Model file for the job. Use its own axes, mm. Face numbers are marked on the shaded views. Give positions to 0.01 mm unless a question says otherwise; leave off trailing zeros. Loops run counter-clockwise (first coordinate to the right, second up) from the corner with the lowest first, then second, coordinate; pieces in that order, holes last. Notation, with made-up numbers: M 36,19 L 94,19 A17 ccw 94,46 Z; hole C 24,63 d3. An arc over 180 degrees is marked long. Answer in a Markdown table with one row per item.
```python
from build123d import *

# Parameters (mm, degrees)
F0_R     = 19.08734
F0_R_2   = 10.668378
F1_DEPTH = 25.4


with BuildPart() as f1:
    # F0 (on Front) → F1 (new body)
    with BuildSketch(Plane.XZ):
        with BuildLine():
            Line((115.265532, 26.16193), (3.586851, 36.99093))
            ThreePointArc((3.586851, 36.99093), (-37.164423, 0), (3.586851, -36.99093))
            Line((3.586851, -36.99093), (115.265532, -26.16193))
            ThreePointArc((115.265532, -26.16193), (139.013356, 0), (115.265532, 26.16193))
        make_face()
        Circle(F0_R, mode=Mode.SUBTRACT)
        with Locations((112.728722, 0)):
            Circle(F0_R_2, mode=Mode.SUBTRACT)
    extrude(amount=F1_DEPTH)


solid = f1.part
```
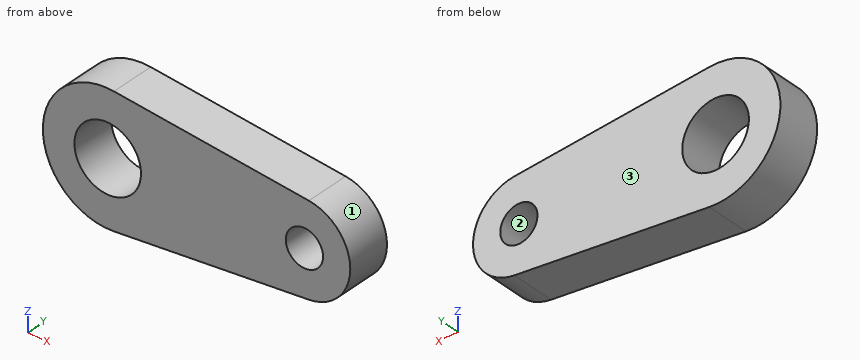
(1) Flat gauge pins, fed straight in: P1, Ø1.5, axis at x = 101, y = -16, coming from the -Z side; P2, Ø5, axis at y = -7, z = 2, coming from the -X side; P3, Ø6, axis at x = 61.5, y = -11.5, coming from the -Z side; P4, Ø6, axis at x = 56.5, y = -5.5, coming from the +Z side. Where does each tip first touch, or does it go through?
Established:
| item | result |
|---|---|
| P1 | stops at z = -27.62 |
| P2 | stops at x = -37.16 |
| P3 | stops at z = -31.67 |
| P4 | stops at z = 32.15 |
(2) Saw through at B-B, the plane z = 0. Give the cut face in (x, y), and give its area (3 significant figures).
Established:
| item | result |
|---|---|
| outline | M -37.16,-25.4 L -19.09,-25.4 L -19.09,0 L -37.16,0 Z; M 19.09,-25.4 L 102.06,-25.4 L 102.06,0 L 19.09,0 Z; M 123.4,-25.4 L 139.01,-25.4 L 139.01,0 L 123.4,0 Z |
| area | 2,960 mm2 |
(3) Saw through at A-A, the plane x = 0. Give the cut face in (y, z).
Established:
| item | result |
|---|---|
| outline | M -25.4,-37.16 L 0,-37.16 L 0,-19.09 L -25.4,-19.09 Z; M -25.4,19.09 L 0,19.09 L 0,37.16 L -25.4,37.16 Z |
(4) Saw through at D-D, the plane x = 111.5. Give the cut face in (y, z), and give its area (3 significant figures).
Established:
| item | result |
|---|---|
| outline | M -25.4,-26.53 L 0,-26.53 L 0,-10.6 L -25.4,-10.6 Z; M -25.4,10.6 L 0,10.6 L 0,26.53 L -25.4,26.53 Z |
| area | 809 mm2 |
(5) Saw through at C-C, the plane y = -7.75. Give the cut face in (x, z).
Established:
| item | result |
|---|---|
| outline | M 3.59,-36.99 L 115.27,-26.16 A26.28 ccw 115.27,26.16 L 3.59,36.99 A37.16 ccw long Z; hole C 0,0 d38.17; hole C 112.73,0 d21.34 |
(6) Mould opens along Z. For the marked faces 1, 2 and 3 say: pulls with the +Z half, pulls with the -Z half, needs draft (parallel to the pull), parting line crosses it, or undercut.
Established:
| item | result |
|---|---|
| face 1 | parting line crosses it |
| face 2 | undercut |
| face 3 | needs draft |
(7) Wall check: L1, parallel to Z at x = 0, y = -19.75; L2, parallel to X at y = -15.75, z = -17; L3, parallel to X at y = -12.5, z = -6.5. Give the ranges that are in metal, low to high.
Established:
| item | result |
|---|---|
| L1 | z = -37.16 to -19.09, 19.09 to 37.16 |
| L2 | x = -33.05 to -8.68, 8.68 to 132.78 |
| L3 | x = -36.59 to -17.95, 17.95 to 104.27, 121.19 to 138.2 |
